Geometry: final body of the model. Coordinates: model frame, mm. Coordinates: 2 decimals unless noted, no trailing zeros. Loops run counter-clockwise (first coordinate to the right, second up) from the corner with the lowest first, then second, coordinate; pieces in that order, holes last. Notation, with made-up numbers: M 21,67.25 L 74,67.25 A18 cw 74,73.25 Z; hole C 89,88.5 d6. An arc over 180 degrees is marked long. Write each question's results on one line, items separated by ' | '. Start each with the question number.
from build123d import *

# Parameters (mm, degrees)
SKETCH2_W                = 38.1
SKETCH2_H                = 38.1
SKETCH2_W_2              = 31.75
SKETCH2_H_2              = 31.75
BOSS_EXTRUDE1_DEPTH      = 381
X_0_397_DIAMETER_HOLE1_D = 10.0838


with BuildPart() as part:
    # Sketch2 → Boss-Extrude1 (new body)
    with BuildSketch(Plane.XY):
        with Locations((19.05, 19.05)):
            Rectangle(SKETCH2_W, SKETCH2_H)
        with Locations((19.05, 19.05)):
            Rectangle(SKETCH2_W_2, SKETCH2_H_2, mode=Mode.SUBTRACT)
    extrude(amount=BOSS_EXTRUDE1_DEPTH)

    # X (0.397) Diameter Hole1 (through all)
    with Locations(Plane.ZY):
        with Locations((19.05, 19.05), (361.95, 19.05)):
            Hole(X_0_397_DIAMETER_HOLE1_D / 2)


solid = part.part
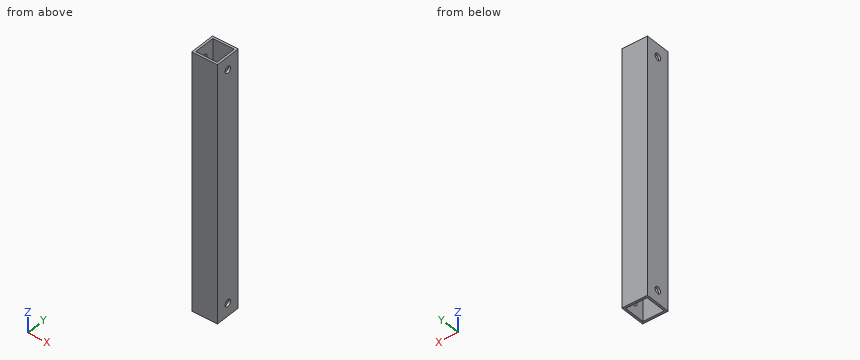
Item 1: Section B-B, the plane z = 361.95. Return loops of the section in (x, y) (3 decimals), plus the area to 3 significant figures.
Item 2: Contact query for a flat-ended pin moving along its axis: P1, Ø8, axis at y = 19.05, z = 19.05, coming from the +X side. Output: stop coordinate, or through.
Item 3: Ray query, L1, parallel to Z at x = 1, y = 19; L2, parallel to X at y = 6, z = 135 (3 decimals); L3, parallel to Y at x = 1.85, z = 361.95. Return the intervals inside material, ascending. Write a range as [from, to].
Item 4: Section A-A, the plane y = 8. Return loops of the section in (x, z) (3 decimals), plus the area to 3 significant figures.
Item 5: Section D-D, the plane z = 79. Return loops of the section in (x, y) (3 decimals), plus the area to 3 significant figures.
Solutions:
1) outline: M 0,0 L 38.1,0 L 38.1,14.008 L 34.925,14.008 L 34.925,3.175 L 3.175,3.175 L 3.175,14.008 L 0,14.008 Z; M 0,24.092 L 3.175,24.092 L 3.175,34.925 L 34.925,34.925 L 34.925,24.092 L 38.1,24.092 L 38.1,38.1 L 0,38.1 Z | area: 380 mm²
2) P1: passes through
3) L1: z = [0, 14.01], [24.09, 356.91], [366.99, 381] | L2: x = [0, 3.175], [34.925, 38.1] | L3: y = [0, 14.01], [24.09, 38.1]
4) outline: M 0,0 L 3.175,0 L 3.175,381 L 0,381 Z; M 34.925,0 L 38.1,0 L 38.1,381 L 34.925,381 Z | area: 2,420 mm²
5) outline: M 0,0 L 38.1,0 L 38.1,38.1 L 0,38.1 Z; hole M 3.175,3.175 L 34.925,3.175 L 34.925,34.925 L 3.175,34.925 Z | area: 444 mm²
